from build123d import *

# Parameters (mm, degrees)
PAD_DEPTH = 2


with BuildPart() as part:
    # Sketch → Pad (new body)
    with BuildSketch(Plane.XY):
        with BuildLine():
            ThreePointArc((235, 0), (217.11169, 89.930607), (166.170094, 166.170094))
            Line((167.230754, 167.230754), (166.170094, 166.170094))
            Line((169.352074, 165.109433), (167.230754, 167.230754))
            Line((170.766288, 166.523647), (169.352074, 165.109433))
            Line((168.644967, 168.644967), (170.766288, 166.523647))
            Line((169.705627, 169.705627), (168.644967, 168.644967))
            ThreePointArc((240, 0), (221.731088, 91.844024), (169.705627, 169.705627))
            Line((240, 0), (238.6, 0))
            Line((238.6, -3.2), (238.6, 0))
            Line((236.4, -3.2), (238.6, -3.2))
            Line((236.4, 0), (236.4, -3.2))
            Line((235, 0), (236.4, 0))
        make_face()
    extrude(amount=PAD_DEPTH)


solid = part.part
The listing builds one solid part. Answer for the finished solid, in the listing's coordinates (mm). Round coordinates to 2 decimals unless told otherwise and drop trailing zeros. Write each loop counter-clockwise with the first axis right and the second up, starting at its lowest first coordinate (ties: lowest second). Pieces come first, ordered by that corner, then holes. Notation, with made-up numbers: M 21.25,54.5 L 47.25,54.5 A31 ccw 47.25,86.5 Z; hole C 76.25,-13 d7. An arc over 180 degrees is marked long. Write each question's results on one line, items separated by ' | '. Start each with the question number.
Item 1: Given pin 1 Ø1 at (y, z) = (-2, 0.5) entering from +X; pin 2 Ø1 at (y, z) = (132, 2) entering from -X; pin 3 Ø5 at (x, y) = (227, 49) entering from -Z; pin 4 Ø1.1 at (x, z) = (235.5, 0.5) entering from -Y, each flat-ended and moving along its own axis, determine where each tip first touches the part or whether it passes through.
Item 2: Find section B-B on x = 183. Write down the section's boundary in (y, z), and give its area (3 significant figures).
Item 3: Find section C-C on y = 127.5. Write down the section's boundary in (x, z), and give its area (3 significant figures).
Item 4: Straight lines are drawn through the part: probe 1 along Y at (x, z) = (170, 0.3); probe 2 along X at (y, z) = (81, 0.8); probe 3 along Y at (x, z) = (173, 0.55). For each, find the intervals that lie inside material, in ascending order.
Item 5: Find section A-A on z = 1.4. Write down the section's boundary in (x, y).
Answer block:
1) pin 1: stops at x = 238.6 | pin 2: stops at x = 194.08 | pin 3: passes through | pin 4: stops at y = 0
2) outline: M 147.43,0 L 155.28,0 L 155.28,2 L 147.43,2 Z | area: 15.7 mm²
3) outline: M 197.41,0 L 203.33,0 L 203.33,2 L 197.41,2 Z | area: 11.9 mm²
4) probe 1: y = 162.25 to 165.76, 167.29 to 169.41 | probe 2: x = 220.6 to 225.92 | probe 3: y = 159.05 to 166.35
5) outline: M 166.17,166.17 A235 cw 235,0 L 236.4,0 L 236.4,-3.2 L 238.6,-3.2 L 238.6,0 L 240,0 A240 ccw 169.71,169.71 L 168.64,168.64 L 170.77,166.52 L 169.35,165.11 L 167.23,167.23 Z
